from build123d import *

# Parameters (mm, degrees)
SKETCH1_R           = 2.575
BOSS_EXTRUDE1_DEPTH = 8.5
SKETCH2_R           = 2.575
SKETCH2_R_2         = 2.45
CUT_EXTRUDE1_DEPTH  = 7.37
FILLET2_R           = 2.45
SKETCH4_R           = 0.2
BOSS_EXTRUDE4_DEPTH = 18
SKETCH6_R           = 0.225
CUT_EXTRUDE2_DEPTH  = 2.5


with BuildPart() as part:
    # Sketch1 → Boss-Extrude1 (new body)
    with BuildSketch(Plane(origin=(0, 0, 0), x_dir=(1, 0, 0), z_dir=(0, 1, 0))):
        Circle(SKETCH1_R)
    extrude(amount=BOSS_EXTRUDE1_DEPTH)

    # Sketch2 → Cut-Extrude1 (cut)
    with BuildSketch(Plane(origin=(0, 8.5, 0), x_dir=(1, 0, 0), z_dir=(0, 1, 0))):
        Circle(SKETCH2_R)
        Circle(SKETCH2_R_2, mode=Mode.SUBTRACT)
    extrude(amount=-CUT_EXTRUDE1_DEPTH, mode=Mode.SUBTRACT)

    # Fillet2
    fillet2_edges = [part.edges().sort_by_distance(p)[0] for p in [
        (-2.45, 8.5, 0),
    ]]
    fillet(fillet2_edges, radius=FILLET2_R)

    # Sketch4 → Boss-Extrude4 (add)
    with BuildSketch(Plane(origin=(0, 0, 0), x_dir=(-1, 0, 0), z_dir=(0, -1, 0))):
        with Locations((1.27, 0)):
            Circle(SKETCH4_R)
        with Locations((-1.27, 0)):
            Circle(SKETCH4_R)
    extrude(amount=BOSS_EXTRUDE4_DEPTH)

    # Sketch6 → Cut-Extrude2 (cut)
    with BuildSketch(Plane.XZ.offset(18)):
        with Locations((1.27, 0)):
            Circle(SKETCH6_R)
    extrude(amount=-CUT_EXTRUDE2_DEPTH, mode=Mode.SUBTRACT)


solid = part.part
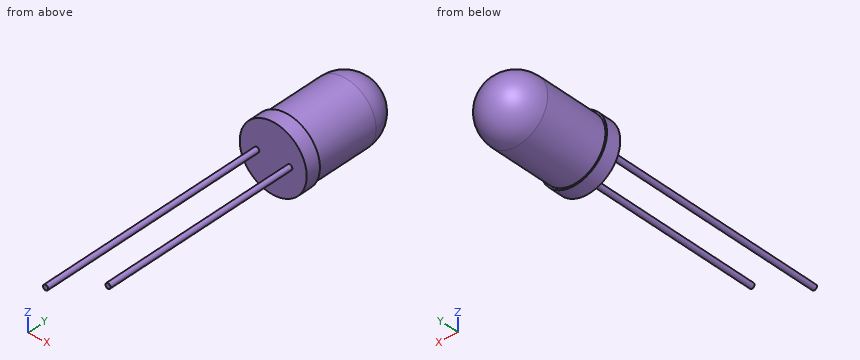
Read the model definition and answer for the solid it produces. Units are mm, in the model's axes. Coordinates: 2 decimals unless noted, no trailing zeros. Loops run counter-clockwise (first coordinate to the right, second up) from the corner with the lowest first, then second, coordinate; pieces in that order, holes last. Notation, with made-up numbers: (22.5, -29.75) -> (73.5, -29.75) arc R4 ccw to (73.5, -24.75) -> close; hole circle Ø1 at (5.5, 79.5). An arc over 180 degrees is marked (long way). Answer in a Markdown table with one row per item.
Item 1: A cutting plane is placed at B-B on y = -12. Determine the outline of the cut face in (x, z), plus the area to 3 significant figures.
Returned:
| item | result |
|---|---|
| outline | circle Ø0.4 at (-1.27, 0); circle Ø0.4 at (1.27, 0) |
| area | 0.251 mm^2 |
Item 2: Straight lines are drawn through the part: line 1 along X through (y, z) = (3, 0.15); line 2 along X through (y, z) = (0.75, 1.35); line 3 along Y through (x, z) = (-0.6, -1). For each, find the intervals that lie inside material, in ascending order. Write a range as [from, to].
Returned:
| item | result |
|---|---|
| line 1 | x = [-2.45, 2.45] |
| line 2 | x = [-2.19, 2.19] |
| line 3 | y = [0, 8.2] |
Item 3: A cutting plane is placed at A-A on x = 0. Determine the outline of the cut face in (y, z) (3 decimals), plus the area to 3 significant figures.
Returned:
| item | result |
|---|---|
| outline | (0, -2.575) -> (1.13, -2.575) -> (1.13, -2.45) -> (6.05, -2.45) arc R2.45 ccw to (6.05, 2.45) -> (1.13, 2.45) -> (1.13, 2.575) -> (0, 2.575) -> close |
| area | 39.4 mm^2 |
Item 4: A cutting plane is placed at D-D on y = 3.5. Determine the outline of the cut face in (x, z).
Returned:
| item | result |
|---|---|
| outline | circle Ø4.9 at (0, 0) |
Item 5: Each of these flat-tipped pins is pushed along its axis until it touches: P1, Ø1, axis at x = 1, z = -2, coming from the +Y side; P2, Ø1.5, axis at x = -0.5, z = -1, coming from the +Y side; P3, Ø1.5, axis at y = 5.5, z = -1, coming from the -X side; P4, Ø1, axis at y = -5.5, z = -2, coming from the -X side. Where does it stop, or does it pass through?
Returned:
| item | result |
|---|---|
| P1 | stops at y = 7.78 |
| P2 | stops at y = 8.47 |
| P3 | stops at x = -2.44 |
| P4 | passes through |
Item 6: A cutting plane is placed at C-C on z = -1.3. Determine the outline of the cut face in (x, y).
Returned:
| item | result |
|---|---|
| outline | (-2.22, 0) -> (2.22, 0) -> (2.22, 1.13) -> (2.08, 1.13) -> (2.08, 6.05) arc R2.08 ccw to (-2.08, 6.05) -> (-2.08, 1.13) -> (-2.22, 1.13) -> close |
